from build123d import *

# Parameters (mm, degrees)
SKETCH_2_R               = 8
CUT_EXTRUDE_1_DEPTH      = 10
SKETCH_3_R               = 1.45
CUT_EXTRUDE_4_DEPTH      = 11
CUT_EXTRUDE_4_DEPTH_BACK = 9
CUT_EXTRUDE_5_REACH      = 8
SKETCH_5_R               = 2.55


with BuildPart() as part:
    # 草图1 → 旋转8 (revolve)
    with BuildSketch(Plane.XY):
        with BuildLine():
            Line((12.68857754, 8), (12.68857754, 0))
            Line((12.68857754, 0), (-15, 0))
            ThreePointArc((-15, 0), (-4.163612428, 14.410563193), (12.68857754, 8))
        make_face()
    revolve(axis=Axis((12.68857754, 0, 0), (-1, 0, 0)))

    # 草图2 → 切除-拉伸1 (cut)
    with BuildSketch(Plane(origin=(12.68857754, 0, 0), x_dir=(0, 0, -1), z_dir=(1, 0, 0))):
        Circle(SKETCH_2_R)
    extrude(amount=-CUT_EXTRUDE_1_DEPTH, mode=Mode.SUBTRACT)

    # 草图3 → 切除-拉伸4 (cut, two sides)
    with BuildSketch(Plane.XY) as cut_extrude_4_sk:
        with Locations((7.68857754, 0)):
            Circle(SKETCH_3_R)
    extrude(amount=CUT_EXTRUDE_4_DEPTH, mode=Mode.SUBTRACT)
    extrude(cut_extrude_4_sk.sketch, amount=-CUT_EXTRUDE_4_DEPTH_BACK, mode=Mode.SUBTRACT)

    # 草图5 → 切除-拉伸5 (cut, up to next)
    with BuildSketch(Plane.XY.offset(-9), mode=Mode.PRIVATE) as cut_extrude_5_sk1:
        with Locations((7.68857754, 0)):
            Circle(SKETCH_5_R)
    cut_extrude_5_tool1 = extrude(cut_extrude_5_sk1.sketch, amount=-CUT_EXTRUDE_5_REACH, mode=Mode.PRIVATE) & part.part
    add(cut_extrude_5_tool1.solids().sort_by_distance((7.688578, 0, -9))[0], mode=Mode.SUBTRACT)


solid = part.part
Source: CAD feature listing. Evaluate the final solid. Frame: model axes, mm. A direction names the side the tool comes from. Give positions to 0.01 mm unless a question says otherwise; leave off trailing zeros. Order: outer loops, then holes, each group sorted by start corner. A loop starts at its lowest first (then second) coordinate and runs counter-clockwise, first axis right, second up. Notation, with made-up numbers: (-11.5, 4.25) -> (25.5, 4.25) arc R27 ccw to (25.5, 43.25) -> close; hole circle Ø5 at (-25, 13). An arc over 180 degrees is marked (long way). Write item = value, one per line.
Q1. Pull-direction query (X, two-part tool) for faces 3 (the face through (2.689, 0, 0)), 4 (the face through (9, -1, -9)), 5 (the face through (8, 0, 11)); classes: released by +X, released by -X, zero draft, split by the parting line, or undercut.
Data:
face_3 = released by +X
face_4 = undercut
face_5 = undercut
Q2. Cut plane D-D, the plane y = 7. Output: boundary loops of the cut face in (x, z), and give its area (3 significant figures).
Data:
outline = (2.69, -3.87) -> (2.69, 3.87) -> (12.69, 3.87) arc R13.27 ccw (long way) to (12.69, -3.87) -> close
area = 472 mm^2
Q3. Cut plane C-C, the plane x = -12.75. Output: boundary loops of the cut face in (y, z), and give its area (3 significant figures).
Data:
outline = circle Ø15.8 at (0, 0)
area = 196 mm^2
Q4. Material intervals for line 1 (Y direction, x = 0.25, z = -0.25); line 2 (X direction, y = 0, z = -10.2); line 3 (X direction, y = 4.5, z = 2.5), sorted ascending. Write a range as from..to.
Data:
line_1 = -15..15
line_2 = -11..5.14, 10.24..11
line_3 = -14.09..2.69
Q5. Set-up query: faces 1 (the face through (7.76, -3.06, -7.39)), 2 (the face through (9.028, -0.555, -8.426)). Return all of +Z, -Z, +X, -X, +Y, -Y with unobstructed straight access to the full face (end or side cutting, diameter ignored); none if empty.
Data:
face_1 = +X
face_2 = -Z
Q6. Pin query (flat end, axial travel): pin 1 (2 mm diameter, centred on y = 4, z = 0, fed in from -X); pin 2 (1.7 mm diameter, centred on x = 7.69, y = 0, fed in from +Z); pin 3 (10 mm diameter, centred on x = 3.5, y = 8, fed in from +Z). Return the tip coordinate at first contact, or that it passes through.
Data:
pin_1 = -14.7
pin_2 = 13.35
pin_3 = 14.53
Q7. Cut plane A-A, the plane y = 0. Output: boundary loops of the cut face in (x, z), and give its area (3 significant figures).
Data:
outline = (2.69, -8) -> (2.69, 8) -> (6.24, 8) -> (6.24, 11) -> (9.14, 11) -> (9.14, 8) -> (12.69, 8) arc R15 ccw (long way) to (5.14, -14.09) -> (5.14, -9) -> (6.24, -9) -> (6.24, -8) -> close; (9.14, -9) -> (10.24, -9) -> (10.24, -10.96) arc R15 ccw to (12.69, -8) -> (9.14, -8) -> close
area = 491 mm^2
Q8. Cut plane B-B, the plane z = 0. Output: boundary loops of the cut face in (x, y).
Data:
outline = (2.69, -8) -> (2.69, 8) -> (12.69, 8) arc R15 ccw (long way) to (12.69, -8) -> close
